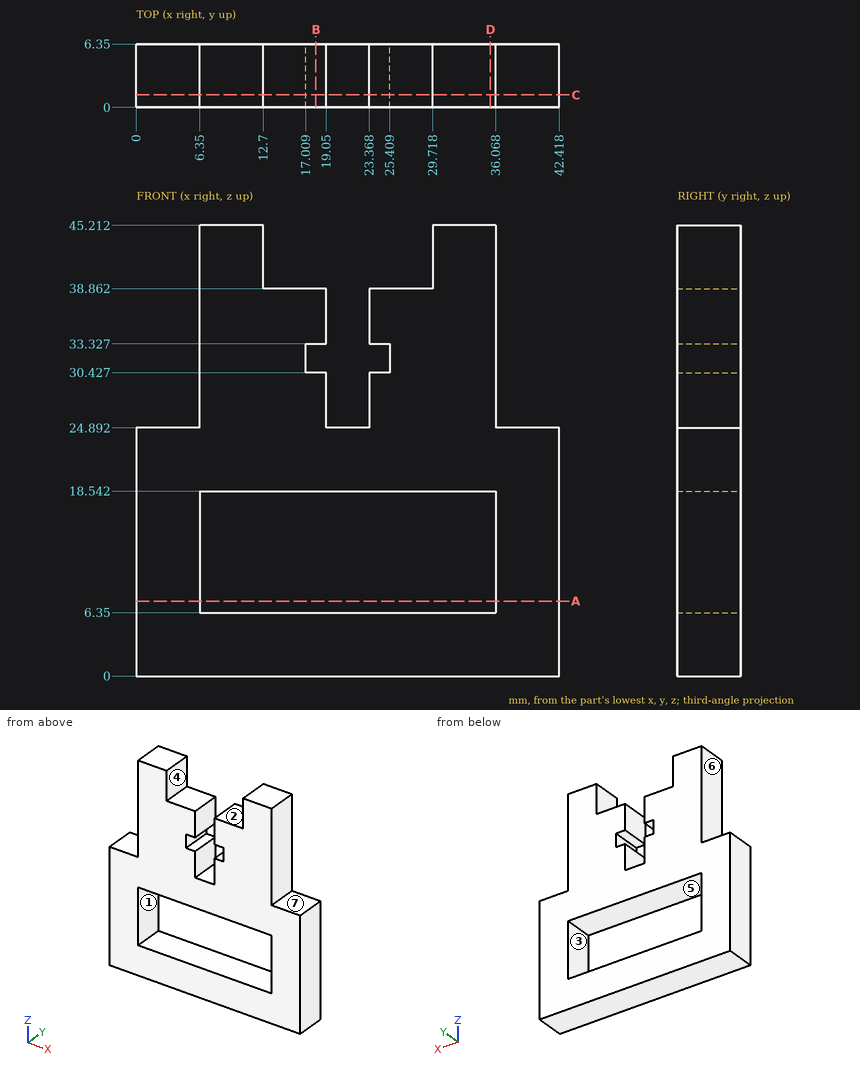
Input: dimensioned drawing with shaded views. Units: mm. Origin: part minimum x, y, z. A direction names the side the tool comes from. Coordinates: 2 decimals unless noted, no trailing zeros. Order: outer loops, then holes, each group sorted by start corner. A loop starts at its lowest first (then second) coordinate and runs counter-clockwise, first axis right, second up.
Item 1: Access query for the marked faces 5, 6 and 7. Directions: +Z, -Z, +X, -X, +Y, -Y. A direction counts if a zero-diameter tool reaches every point of the face in a straight line with its end or side. Return the directions, or none.
Answer:
face 5: +Y, -Y
face 6: +Z, -X, +Y, -Y
face 7: +Z, +X, +Y, -Y
Item 2: Draft query along Z for the marked faces 1, 2, 3 and 4. Return one class per face: released by +Z, released by -Z, zero draft, split by the parting line, or undercut.
Answer:
face 1: undercut
face 2: released by +Z
face 3: undercut
face 4: zero draft
Item 3: Section query C-C (y = 1.25). Output: boundary loops of the cut face in (x, z), then the cut area to 3 significant figures.
Answer:
outline: (0, 0) - (42.42, 0) - (42.42, 24.89) - (36.07, 24.89) - (36.07, 45.21) - (29.72, 45.21) - (29.72, 38.86) - (23.37, 38.86) - (23.37, 33.33) - (25.41, 33.33) - (25.41, 30.43) - (23.37, 30.43) - (23.37, 24.89) - (19.05, 24.89) - (19.05, 30.43) - (17.01, 30.43) - (17.01, 33.33) - (19.05, 33.33) - (19.05, 38.86) - (12.7, 38.86) - (12.7, 45.21) - (6.35, 45.21) - (6.35, 24.89) - (0, 24.89) - close; hole (6.35, 6.35) - (36.07, 6.35) - (36.07, 18.54) - (6.35, 18.54) - close
area: 1,120 mm2
Item 4: Section query A-A (z = 7.5). Output: boundary loops of the cut face in (x, y).
Answer:
outline: (0, 0) - (6.35, 0) - (6.35, 6.35) - (0, 6.35) - close; (36.07, 0) - (42.42, 0) - (42.42, 6.35) - (36.07, 6.35) - close
Item 5: Material intervals for line 1 along X through (y, z) = (3, 7.5); line 2 along X through (y, z) = (4, 35); line 3 along Z through (x, y) = (25.5, 5.25), sorted ascending.
Answer:
line 1: x = 0 to 6.35, 36.07 to 42.42
line 2: x = 6.35 to 19.05, 23.37 to 36.07
line 3: z = 0 to 6.35, 18.54 to 38.86
Item 6: Section query D-D (x = 35.5). Output: boundary loops of the cut face in (y, z), then the cut area to 3 significant figures.
Answer:
outline: (0, 0) - (6.35, 0) - (6.35, 6.35) - (0, 6.35) - close; (0, 18.54) - (6.35, 18.54) - (6.35, 45.21) - (0, 45.21) - close
area: 210 mm2
Item 7: Section query B-B (x = 18). Output: boundary loops of the cut face in (y, z), then the cut area to 3 significant figures.
Answer:
outline: (0, 0) - (6.35, 0) - (6.35, 6.35) - (0, 6.35) - close; (0, 18.54) - (6.35, 18.54) - (6.35, 30.43) - (0, 30.43) - close; (0, 33.33) - (6.35, 33.33) - (6.35, 38.86) - (0, 38.86) - close
area: 151 mm2
Item 8: Contact query for flat-ended pins moving along their axis: P1, Ø2, axis at x = 24.5, y = 2, coming from the +Z side; P2, Ø2, axis at x = 20.5, y = 2, coming from the +Z side; P3, Ø1.5, axis at y = 4, z = 32, coming from the -X side. Output: stop coordinate, or through.
Answer:
P1: stops at z = 38.86
P2: stops at z = 24.89
P3: stops at x = 6.35
